Work out the finished part from the listing and answer in its coordinate system (mm). A direction names the side the tool comes from. Coordinates: 2 decimals unless noted, no trailing zeros. Order: outer loops, then holes, each group sorted by start corner. A loop starts at its lowest first (then second) coordinate and runs counter-clockwise, first axis right, second up.
1. The part is cut by section A-A, the plane x = 0. Give the vertices of the cut face in (y, z).
2. The part is cut by section B-B, the plane z = -154. Give the vertices of the cut face in (x, y) (3 decimals), then the cut area to 3 significant figures.
3. The part is cut by section D-D, the plane y = 23. Give the vertices of the cut face in (x, z).
4. The part is cut by section C-C, the plane z = -121.5. Give the vertices of the cut face in (x, y) (3 decimals), then the cut area to 3 significant figures.
5. Determine the mould class of faces 4 (the flat face through (-10, 6, -139)), 5 (the flat face through (9, 39, -127)), 6 (the flat face through (13, -1.427, -139)) for opening direction Y: +Y half, -Y half, draft (parallel to the pull), parting line (faces both ways), or undercut.
6. Flat-ended cylindrical pins translate along their axes: pin 1 Ø20.5 at (x, z) = (-3, -112.5) entering from +Y; pin 2 Ø2 at (y, z) = (17, -122.5) entering from +X; pin 3 Ø1.5 at (y, z) = (34, -133) entering from -X; pin 4 Ø1.5 at (y, z) = (16, -117) entering from -X. Find the tip coordinate at first contact, or state that the pin passes through.
7. A tool of negligible diameter and unlimited length cuts with its end or side. For faces 1 (the cylindrical face through (18.095, 14.979, -114.478)), 2 (the flat face through (0, 15.884, -114)), 3 (the flat face through (7.274, 0, -139)), from which of +Z, -Z, +X, -X, +Y, -Y can it reach the whole face along a straight path? Write none if from no direction.
8. Find the intervals of material crossed by probe 1 along Y at (x, z) = (0, -149); probe 2 along Y at (x, z) = (8, -148.5); probe 3 along Z at (x, y) = (5, 16), in increasing order.
Autodesk Inventor part; units mm, degrees
ref_plane "YZ Plane" through (0, 0, 0) normal (1, 0, 0) x (0, 1, 0)
ref_plane "XZ Plane" through (0, 0, 0) normal (0, 1, 0) x (-1, 0, 0)
ref_plane "XY Plane" through (0, 0, 0) normal (0, 0, 1) x (1, 0, 0)
sketch "Sketch1" plane through (0, 0, 0) normal (0, 0, 1) x (1, 0, 0)
  line L0 (-7.2739, -1.4271) -> (7.2739, -1.4271)
  line L1 (7.2739, -1.4271) -> (7.2739, 1.4271)
  line L2 (7.2739, 1.4271) -> (-7.2739, 1.4271)
  line L3 (-7.2739, 1.4271) -> (-7.2739, -1.4271)
  line L4 (-7.2739, -1.4271) -> (7.2739, 1.4271) construction
  line L5 (7.2739, -1.4271) -> (-7.2739, 1.4271) construction
  line L6 (9.525, 3.6783) -> (-9.525, 3.6783)
  line L7 (-9.525, 3.6783) -> (-9.525, 6.4723)
  line L8 (-9.525, 6.4723) -> (9.525, 6.4723)
  line L9 (9.525, 6.4723) -> (9.525, 3.6783)
  line L10 (9.525, 3.6783) -> (-9.525, 6.4723) construction
  line L11 (-9.525, 3.6783) -> (9.525, 6.4723) construction
  line L12 (-7.2739, 1.4271) -> (-9.525, 3.6783)
  line L13 (7.2739, 1.4271) -> (9.525, 3.6783)
  line L14 (-10.922, 5.0753) -> (-8.1026, 7.8947)
  line L15 (-10.922, 5.0753) -> (-6.9348, 5.0753) construction
  line L16 (-10.922, 5.0753) -> (-9.525, 3.6783)
  line L17 (10.922, 5.0753) -> (8.1026, 7.8947)
  line L18 (9.525, 3.6783) -> (10.922, 5.0753)
  line L19 (-8.1026, 7.8947) -> (8.1026, 7.8947)
  line L20 (-19.05, -1.4271) -> (19.05, -1.4271)
  line L21 (19.05, -1.4271) -> (19.05, 15.8839)
  line L22 (19.05, 15.8839) -> (-19.05, 15.8839)
  line L23 (-19.05, 15.8839) -> (-19.05, -1.4271)
  point P0 (0, 0)
  point P1 (0, 5.0753)
  point P2 (0, -1.4271)
  dimension "d0" = 135
  dimension "d1" = 135
  dimension "d2" = 19.05
  dimension "d3" = 2.794
  dimension "d4" = 45
  dimension "d5" = 4.2164
  dimension "d6" = 90
  dimension "d7" = 90
  dimension "d8" = 9.3218
  dimension "d9" = 38.1
extrude "Extrusion1" add sketch "Sketch1" against normal blind 177.8 contours L20 L23 L22 L21 L1 L13 L18 L17 L19 L14 L16 L12 L3
sketch "Sketch2" plane through (0, 0, -177.8) normal (0, 0, -1) x (-1, 0, 0)
  arc A0 (19.05, 29.7163) -> (-19.05, 29.7163) centre (0, 29.7163) ccw
  line L0 (19.05, -1.4271) -> (19.05, 15.8839)
  line L1 (19.05, 15.8839) -> (19.05, -1.4271)
  line L2 (19.05, 15.8839) -> (19.05, 29.7163)
  line L3 (-19.05, -1.4271) -> (-19.05, 15.8839)
  line L4 (-19.05, 15.8839) -> (-19.05, 29.7163)
  line L5 (19.05, 15.8839) -> (-19.05, 15.8839)
  point P0 (0, 0)
extrude "Extrusion2" add sketch "Sketch2" against normal blind 50.8
sketch "Sketch3" plane through (0, 0, -177.8) normal (0, 0, -1) x (-1, 0, 0)
  arc A0 (19.05, 29.7163) -> (-19.05, 29.7163) centre (0, 29.7163) ccw
  point P0 (0, 0)
hole "Hole1" at (0, 29.7163, -177.8) direction (0, 0, 1) diameter 21.6 end through all
fillet "Fillet1" radius 3.175 2 edges at (-19.05, 15.8839, -63.5) (19.05, 15.8839, -63.5)
sketch "Sketch4" plane through (0, 0, 0) normal (0, 0, 1) x (1, 0, 0)
  line L0 (-84.0587, 46.9015) -> (30.6415, 46.9015)
  line L1 (30.6415, 46.9015) -> (30.6415, -6.8679)
  line L2 (30.6415, -6.8679) -> (-84.0587, -6.8679)
  line L3 (-84.0587, -6.8679) -> (-84.0587, 46.9015)
  line L4 (-84.0587, 46.9015) -> (30.6415, -6.8679) construction
  line L5 (30.6415, 46.9015) -> (-84.0587, -6.8679) construction
  point P0 (0, 0)
  point P1 (-26.7086, 20.0168)
extrude "Extrusion3" cut sketch "Sketch4" against normal blind 101.6
properties part number "Laser mount 3 inches"
Geometry says:
1. outline: (7.89, -177.8) - (18.92, -177.8) - (18.92, -127) - (15.88, -127) - (15.88, -101.6) - (7.89, -101.6) - close; (40.52, -177.8) - (48.77, -177.8) - (48.77, -127) - (40.52, -127) - close
2. outline: (-19.05, -1.427) - (-7.274, -1.427) - (-7.274, 1.427) - (-9.525, 3.678) - (-10.922, 5.075) - (-8.103, 7.895) - (8.103, 7.895) - (10.922, 5.075) - (9.525, 3.678) - (7.274, 1.427) - (7.274, -1.427) - (19.05, -1.427) - (19.05, 29.716) arc R19.05 ccw to (-19.05, 29.716) - close; hole circle Ø21.6 at (0, 29.716)
2. area: 1,230 mm2
3. outline: (-19.05, -177.8) - (-8.46, -177.8) - (-8.46, -127) - (-19.05, -127) - close; (8.46, -177.8) - (19.05, -177.8) - (19.05, -127) - (8.46, -127) - close
4. outline: (-19.05, -1.427) - (-7.274, -1.427) - (-7.274, 1.427) - (-9.525, 3.678) - (-10.922, 5.075) - (-8.103, 7.895) - (8.103, 7.895) - (10.922, 5.075) - (9.525, 3.678) - (7.274, 1.427) - (7.274, -1.427) - (19.05, -1.427) - (19.05, 12.709) arc R3.175 ccw to (15.875, 15.884) - (-15.875, 15.884) arc R3.175 ccw to (-19.05, 12.709) - close
4. area: 494 mm2
5. face 4: undercut
5. face 5: draft
5. face 6: -Y half
6. pin 1: stops at y = 15.88
6. pin 2: passes through
6. pin 3: stops at x = -18.72
6. pin 4: stops at x = -17.78
7. face 1: +Z, +X, +Y
7. face 2: +Z, +X, -X, +Y
7. face 3: +Z, -Z, -Y
8. probe 1: y = 7.89 to 18.92, 40.52 to 48.77
8. probe 2: y = -1.43 to 2.15, 7.89 to 22.46, 36.97 to 47.01
8. probe 3: z = -177.8 to -127
